Work out the finished part from the listing and answer in its coordinate system (mm). Face numbers are marked on the shaded views. A direction names the side the tool comes from. Give positions to 0.01 mm unless a question says otherwise; leave off trailing zeros. Loops run counter-clockwise (first coordinate to the right, second up) from the corner with the lowest first, then second, coordinate; pieces in that order, holes last. Notation, with made-up numbers: M 88.25,3.5 L 102.25,3.5 A20 ccw 102.25,17.5 Z; hole C 43,-12 d1. An arc over 180 degrees is marked long. Use a Markdown table: item, result.
```python
from build123d import *

# Parameters (mm, degrees)
F0_R     = 17.819723
F1_DEPTH = 72.898


with BuildPart() as f1:
    # F0 (on Top) → F1 (new body)
    with BuildSketch(Plane.XY):
        Polygon((16.365739, 42.712353), (16.365739, 58.036424), (0, 58.036424), (0, 47.588196), (-10.799658, 47.588196), (-10.799658, 35.050321), (-23.685807, 35.050321), (-23.685807, 22.860721), (-32.044392, 22.860721), (-32.044392, 34.0055), (-50.154656, 34.0055), (-50.154656, 18.681431), (-36.223684, 18.681431), (-36.223684, 8.581474), (-50.50293, 8.581474), (-50.50293, 0.048754), (-59.906334, 0.048754), (-59.906334, -15.797727), (-46.323638, -15.797727), (-46.323638, -8.483966), (-32.740939, -8.483966), (-32.740939, 4.402183), (-24.034083, 4.402183), (-24.034083, -10.892829), (-10.797826, -10.892829), (-10.103109, 7.536652), (-20.203065, 7.536652), (-20.203065, 18.333156), (-10.103109, 18.333156), (-6.272093, 18.333156), (-6.272093, 30.174481), (4.524411, 30.174481), (4.524411, 42.712353), align=None)
        with BuildLine():
            Line((-7.66519, -10.892829), (-10.797826, -10.892829))
            Line((-10.797826, -10.892829), (-24.034083, -10.892829))
            Line((-24.034083, -10.892829), (-28.387511, -10.892829))
            Line((-28.387511, -10.892829), (-28.387511, -46.7868))
            Line((-28.387511, -46.7868), (-28.387511, -51.6636))
            Line((-28.387511, -51.6636), (68.580002, -51.6636))
            Line((68.580002, -51.6636), (68.795034, -49.802116))
            ThreePointArc((68.795034, -49.802116), (59.54773, -49.482859), (51.229698, -45.430098))
            Line((51.229698, -45.430098), (10.961137, -45.430098))
            Line((10.961137, -45.430098), (4.253947, -45.430098))
            Line((4.253947, -45.430098), (-7.66519, -45.430098))
            Line((-7.66519, -45.430098), (-24.034083, -45.430098))
            Line((-24.034083, -45.430098), (-24.034083, -19.541675))
            Line((-24.034083, -19.541675), (-15.543758, -19.541675))
            Line((-15.543758, -19.541675), (-15.543758, -32.4612))
            Line((-15.543758, -32.4612), (-15.543758, -37.642799))
            Line((-15.543758, -37.642799), (8.223667, -37.360428))
            Line((8.223667, -37.360428), (14.522387, -37.285595))
            Line((14.522387, -37.285595), (44.588531, -36.928391))
            ThreePointArc((44.588531, -36.928391), (43.183524, -32.642564), (42.671578, -28.161463))
            Line((42.671578, -28.161463), (-7.66519, -28.161463))
            Line((-7.66519, -28.161463), (-7.66519, -10.892829))
        make_face()
        with BuildLine():
            ThreePointArc((87.174887, -27.8892), (64.786265, -5.637128), (42.671578, -28.161463))
            ThreePointArc((42.671578, -28.161463), (43.183524, -32.642564), (44.588531, -36.928391))
            ThreePointArc((44.588531, -36.928391), (47.386105, -41.587797), (51.229698, -45.430098))
            ThreePointArc((51.229698, -45.430098), (59.54773, -49.482859), (68.795034, -49.802116))
            ThreePointArc((68.795034, -49.802116), (81.971578, -42.189505), (87.174887, -27.8892))
        make_face()
        with Locations((64.9224, -27.8892)):
            Circle(F0_R, mode=Mode.SUBTRACT)
        Polygon((10.961137, -45.430098), (14.522387, -37.285595), (8.223667, -37.360428), (4.253947, -45.430098), align=None)
    extrude(amount=F1_DEPTH)


solid = f1.part
```
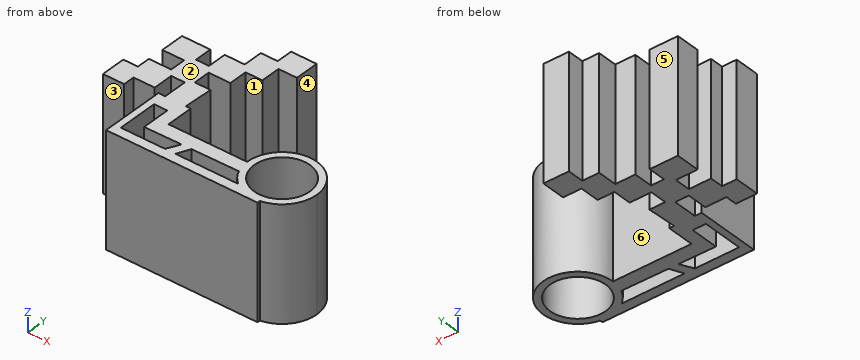
(1) Which of the six approach directions +Z, -Z, +X, -X, +Y, -Y give full straight-line access (tool end or side, diameter ignored) to the marked faces 4, 5 and 6?
Entries:
| item | result |
|---|---|
| face 4 | +Z, -Z, +X, +Y |
| face 5 | +Z, -Z, -X, +Y |
| face 6 | +Z, -Z |
(2) A cutting plane is placed at D-D (y = -22). Write down the section's boundary in (x, z).
Entries:
| item | result |
|---|---|
| outline | M -28.39,0 L -24.03,0 L -24.03,72.9 L -28.39,72.9 Z; M -15.54,0 L -7.67,0 L -7.67,72.9 L -15.54,72.9 Z; M 43.46,0 L 48.1,0 L 48.1,72.9 L 43.46,72.9 Z; M 81.74,0 L 86.38,0 L 86.38,72.9 L 81.74,72.9 Z |
(3) A cutting plane is placed at A-A (y = -35). Write down the section's boundary in (x, z), and give its area (3 significant figures).
Entries:
| item | result |
|---|---|
| outline | M -28.39,0 L -24.03,0 L -24.03,72.9 L -28.39,72.9 Z; M -15.54,0 L 48.58,0 L 48.58,72.9 L -15.54,72.9 Z; M 81.26,0 L 86.01,0 L 86.01,72.9 L 81.26,72.9 Z |
| area | 5,340 mm² |
(4) A cutting plane is placed at B-B (x = 61). Write down the section's boundary in (y, z), and give its area (3 significant figures).
Entries:
| item | result |
|---|---|
| outline | M -51.66,0 L -45.27,0 L -45.27,72.9 L -51.66,72.9 Z; M -10.51,0 L -5.99,0 L -5.99,72.9 L -10.51,72.9 Z |
| area | 796 mm² |
(5) Given P1, Ø8.5, axis at y = 51, z = 31.5, coming from the -X side; P2, Ø7, axis at x = -42.5, z = 42, coming from the +Y side; P3, Ø17, axis at y = 48, z = 19, coming from the +X side; P4, Ø1, axis at x = -12, y = 10, coming from the -Z side, each flat-ended and moving along its own axis, determine where each tip first touches the part or whether it passes through.
Entries:
| item | result |
|---|---|
| P1 | stops at x = -10.8 |
| P2 | stops at y = 34.01 |
| P3 | stops at x = 16.37 |
| P4 | passes through |
(6) Consider probe 1 along Y at (x, z) = (42.5, 12); probe 2 along X at (y, z) = (25, 20.5); probe 3 along Y at (x, z) = (-4, 11). Determine where each line is inside the solid, lowest interval first. Write a range as [from, to].
Entries:
| item | result |
|---|---|
| probe 1 | y = [-51.66, -45.43], [-36.95, -28.16] |
| probe 2 | x = [-50.15, -32.04], [-23.69, -6.27] |
| probe 3 | y = [-51.66, -45.43], [-37.51, -28.16], [30.17, 47.59] |
(7) A cutting plane is placed at C-C (z = 27.5). Count the separate pieces of the cut face and the enclosed holes in it, and give its area (3 significant figures).
Entries:
| item | result |
|---|---|
| separate pieces | 1 |
| enclosed holes | 3 |
| area | 4,060 mm² |
(8) The mould has two halves that part along Y. Classify the marked faces 1, 2 and 3: released by +Y, released by -Y, zero draft, split by the parting line, or undercut.
Entries:
| item | result |
|---|---|
| face 1 | undercut |
| face 2 | zero draft |
| face 3 | released by -Y |
